```python
from build123d import *

# Parameters (mm, degrees)
BOX003_W                    = 40
BOX003_H                    = 40
BOX003_DEPTH                = 10
CYLINDER014_R               = 10.2
CYLINDER014_DEPTH           = 20
CYLINDER014_ROLL_ANGLE      = 7.107076
CYLINDER014_PITCH_ANGLE     = 7.053022
CYLINDER014_PLACEMENT_ANGLE = 0.438549
CYLINDER013_R               = 10.2
CYLINDER013_DEPTH           = 20
CYLINDER013_ROLL_ANGLE      = 3.540025
CYLINDER013_PITCH_ANGLE     = 3.533287
CYLINDER013_PLACEMENT_ANGLE = 0.109222
CYLINDER012_R               = 10.2
CYLINDER012_DEPTH           = 20
CYLINDER011_R               = 10.2
CYLINDER011_DEPTH           = 20
CYLINDER011_ROLL_ANGLE      = -3.540025
CYLINDER011_PITCH_ANGLE     = -3.533287
CYLINDER011_PLACEMENT_ANGLE = 0.109222
CYLINDER010_R               = 10.2
CYLINDER010_DEPTH           = 20
CYLINDER010_ROLL_ANGLE      = -7.107076
CYLINDER010_PITCH_ANGLE     = -7.053022
CYLINDER010_PLACEMENT_ANGLE = 0.438549
BOX002_W                    = 116
BOX002_H                    = 32
BOX002_DEPTH                = 14
BOX002_PITCH_ANGLE          = 10
BOX001_W                    = 116
BOX001_H                    = 32
BOX001_DEPTH                = 14
BOX001_PITCH_ANGLE          = -10
BOX_W                       = 116
BOX_H                       = 32
BOX_DEPTH                   = 20
CHAMFER_SIZE                = 4


with BuildPart() as cube003:
    # Box003 → Box003 (new body)
    with BuildSketch(Plane(origin=(20, -20, 10.3), x_dir=(1, 0, 0), z_dir=(0, 0, 1))):
        with Locations((20, 20)):
            Rectangle(BOX003_W, BOX003_H)
    extrude(amount=BOX003_DEPTH)


with BuildPart() as cylinder014:
    # Cylinder014 → Cylinder014 (new body)
    with BuildSketch(Plane.XY):
        Circle(CYLINDER014_R)
    extrude(amount=CYLINDER014_DEPTH)


with BuildPart() as cylinder014_1:
    # Cylinder014 roll: moved
    add(cylinder014.part.rotate(Axis((0, 0, 0), (1, 0, 0)), CYLINDER014_ROLL_ANGLE))


with BuildPart() as cylinder014_2:
    # Cylinder014 pitch: moved
    add(cylinder014_1.part.rotate(Axis((0, 0, 0), (0, 1, 0)), CYLINDER014_PITCH_ANGLE))


with BuildPart() as cylinder014_3:
    # Cylinder014 placement: moved
    add(cylinder014_2.part.moved(Location((84, 0, -4))).rotate(Axis((84, 0, -4), (0, 0, 1)), CYLINDER014_PLACEMENT_ANGLE))


with BuildPart() as cylinder013:
    # Cylinder013 → Cylinder013 (new body)
    with BuildSketch(Plane.XY):
        Circle(CYLINDER013_R)
    extrude(amount=CYLINDER013_DEPTH)


with BuildPart() as cylinder013_1:
    # Cylinder013 roll: moved
    add(cylinder013.part.rotate(Axis((0, 0, 0), (1, 0, 0)), CYLINDER013_ROLL_ANGLE))


with BuildPart() as cylinder013_2:
    # Cylinder013 pitch: moved
    add(cylinder013_1.part.rotate(Axis((0, 0, 0), (0, 1, 0)), CYLINDER013_PITCH_ANGLE))


with BuildPart() as cylinder013_3:
    # Cylinder013 placement: moved
    add(cylinder013_2.part.moved(Location((63, 0, -1))).rotate(Axis((63, 0, -1), (0, 0, 1)), CYLINDER013_PLACEMENT_ANGLE))


with BuildPart() as cylinder012:
    # Cylinder012 → Cylinder012 (new body)
    with BuildSketch(Plane(origin=(41.7, 0, 0), x_dir=(1, 0, 0), z_dir=(0, 0, 1))):
        Circle(CYLINDER012_R)
    extrude(amount=CYLINDER012_DEPTH)


with BuildPart() as cylinder011:
    # Cylinder011 → Cylinder011 (new body)
    with BuildSketch(Plane.XY):
        Circle(CYLINDER011_R)
    extrude(amount=CYLINDER011_DEPTH)


with BuildPart() as cylinder011_1:
    # Cylinder011 roll: moved
    add(cylinder011.part.rotate(Axis((0, 0, 0), (1, 0, 0)), CYLINDER011_ROLL_ANGLE))


with BuildPart() as cylinder011_2:
    # Cylinder011 pitch: moved
    add(cylinder011_1.part.rotate(Axis((0, 0, 0), (0, 1, 0)), CYLINDER011_PITCH_ANGLE))


with BuildPart() as cylinder011_3:
    # Cylinder011 placement: moved
    add(cylinder011_2.part.moved(Location((21, 0, -1))).rotate(Axis((21, 0, -1), (0, 0, 1)), CYLINDER011_PLACEMENT_ANGLE))


with BuildPart() as cylinder010:
    # Cylinder010 → Cylinder010 (new body)
    with BuildSketch(Plane.XY):
        Circle(CYLINDER010_R)
    extrude(amount=CYLINDER010_DEPTH)


with BuildPart() as cylinder010_1:
    # Cylinder010 roll: moved
    add(cylinder010.part.rotate(Axis((0, 0, 0), (1, 0, 0)), CYLINDER010_ROLL_ANGLE))


with BuildPart() as cylinder010_2:
    # Cylinder010 pitch: moved
    add(cylinder010_1.part.rotate(Axis((0, 0, 0), (0, 1, 0)), CYLINDER010_PITCH_ANGLE))


with BuildPart() as cylinder010_3:
    # Cylinder010 placement: moved
    add(cylinder010_2.part.moved(Location((0, 0, -4))).rotate(Axis((0, 0, -4), (0, 0, 1)), CYLINDER010_PLACEMENT_ANGLE))


with BuildPart() as cube002:
    # Box002 → Box002 (new body)
    with BuildSketch(Plane.XY):
        with Locations((58, 16)):
            Rectangle(BOX002_W, BOX002_H)
    extrude(amount=BOX002_DEPTH)


with BuildPart() as cube002_1:
    # Box002 pitch: moved
    add(cube002.part.rotate(Axis((0, 0, 0), (0, 1, 0)), BOX002_PITCH_ANGLE))


with BuildPart() as cube002_2:
    # Box002 placement: moved
    add(cube002_1.part.moved(Location((0, -16, 19.5))))


with BuildPart() as cube001:
    # Box001 → Box001 (new body)
    with BuildSketch(Plane.XY):
        with Locations((58, 16)):
            Rectangle(BOX001_W, BOX001_H)
    extrude(amount=BOX001_DEPTH)


with BuildPart() as cube001_1:
    # Box001 pitch: moved
    add(cube001.part.rotate(Axis((0, 0, 0), (0, 1, 0)), BOX001_PITCH_ANGLE))


with BuildPart() as cube001_2:
    # Box001 placement: moved
    add(cube001_1.part.moved(Location((-30, -16, -0.5))))


with BuildPart() as cut011:
    # Box → Box (new body)
    with BuildSketch(Plane(origin=(-16, -16, -7), x_dir=(1, 0, 0), z_dir=(0, 0, 1))):
        with Locations((58, 16)):
            Rectangle(BOX_W, BOX_H)
    extrude(amount=BOX_DEPTH)

    # Cut005: cut Cube001
    add(cube001_2.part, mode=Mode.SUBTRACT)

    # Cut006: cut Cube002
    add(cube002_2.part, mode=Mode.SUBTRACT)

    # Chamfer
    chamfer_edges = [cut011.edges().sort_by_distance(p)[0] for p in [
        (-16, -16, -2.515711),
        (-16, 0, 1.968578),
        (-16, 16, -2.515711),
        (100, -16, -2.566349),
        (70.856409, -16, 7.006103),
        (12.856409, -16, 7.056741),
        (12.856409, 16, 7.056741),
        (100, 16, -2.566349),
        (70.856409, 16, 7.006103),
        (100, 0, 1.867302),
    ]]
    chamfer(chamfer_edges, length=CHAMFER_SIZE)

    # Cut: cut Cylinder010
    add(cylinder010_3.part, mode=Mode.SUBTRACT)

    # Cut007: cut Cylinder011
    add(cylinder011_3.part, mode=Mode.SUBTRACT)

    # Cut008: cut Cylinder012
    add(cylinder012.part, mode=Mode.SUBTRACT)

    # Cut009: cut Cylinder013
    add(cylinder013_3.part, mode=Mode.SUBTRACT)

    # Cut010: cut Cylinder014
    add(cylinder014_3.part, mode=Mode.SUBTRACT)

    # Cut011: cut Cube003
    add(cube003.part, mode=Mode.SUBTRACT)


solid = cut011.part
```
Work out the finished part from the listing and answer in its coordinate system (mm). A direction names the side the tool comes from. Give positions to 0.01 mm unless a question says otherwise; leave off trailing zeros. Order: outer loops, then holes, each group sorted by start corner. A loop starts at its lowest first (then second) coordinate and runs counter-clockwise, first axis right, second up. Notation, with made-up numbers: (42, 69.5) - (57, 69.5) arc R22 ccw to (57, 86.5) - close; hole circle Ø4 at (33, 42). An arc over 180 degrees is marked (long way). One line per item, written item: value. Start each with the question number.
1. Consider line 1 (X direction, y = 1, z = 1); line 2 (Y direction, x = 41.7, z = 7); line 3 (X direction, y = 7.5, z = 1.5). Determine where each line is inside the solid, lowest interval first.
2. Each of these flat-tipped pins is pushed along its axis until it touches: pin 1 Ø10 at (y, z) = (-7, 0) entering from +X; pin 2 Ø6 at (y, z) = (7.5, 1) entering from -X; pin 3 Ø1 at (y, z) = (11.5, 1.5) entering from -X; pin 4 Ø1 at (y, z) = (3.5, 8) entering from -X. Where does it stop, or does it pass through?
3. Which of the six approach directions +Z, -Z, +X, -X, +Y, -Y give full straight-line access (tool end or side, diameter ignored) to faces 4 (the face through (42, 0, 0)), 5 (the face through (14.325, -14.028, 5.256))?
4. For a pull along Z with two mould halves and no side action, classify faces 1 (the face through (55.16, -6.46, 3.19)), 2 (the face through (73.811, 2.835, 6.485)), 3 (the face through (-14, 14, -4)) as released by +Z, released by -Z, zero draft, split by the parting line, or undercut.
5. Section A-A, the plane x = 48 is taken. Write down the section's boundary in (y, z), then the cut area to 3 significant figures.
Filled sheet:
1. line 1: -13.46 to -10.9, 9.64 to 10.69, 31.05 to 31.55, 51.85 to 52.96, 73.28 to 74.45, 94.75 to 97.37
1. line 2: -16 to -10.2, 10.2 to 16
1. line 3: -13.04 to -8.48, 6.9 to 13.71, 27.92 to 34.79, 48.61 to 56.35, 69.9 to 78.34, 90.78 to 96.95
2. pin 1: x = 100
2. pin 2: x = -15.97
2. pin 3: x = -13.46
2. pin 4: x = 30.05
3. face 4: +Z
3. face 5: +Z, -X, -Y
4. face 1: undercut
4. face 2: released by +Z
4. face 3: zero draft
5. outline: (-16, -7) - (16, -7) - (16, 6.97) - (12.73, 10.3) - (8.02, 10.3) - (8.02, 0) - (-8.02, 0) - (-8.02, 10.3) - (-12.73, 10.3) - (-16, 6.97) - close
5. area: 377 mm²
